from build123d import *

# Parameters (mm, degrees)
SZKIC2_R                   = 2.5
WYTNIJ_WYCI_GNI_CIE1_DEPTH = 102.105666205
ZAOKR_GLENIE1_R            = 10
ZAOKR_GLENIE2_R            = 5
SFAZOWANIE1_SIZE           = 1
SFAZOWANIE2_SIZE           = 0.5
SFAZOWANIE3_SIZE           = 0.5
SZKIC3_R                   = 8
WYTNIJ_WYCI_GNI_CIE2_DEPTH = 100.811551129


with BuildPart() as part:
    # Szkic1 → Obrót1 (revolve)
    with BuildSketch(Plane.XY, mode=Mode.PRIVATE) as obr_t1_sk:
        with BuildLine():
            Line((0, 27.578244749), (0, 21.078244749))
            Line((0, 21.078244749), (-8, 21.078244749))
            Line((-8, 21.078244749), (-8, -8.921755251))
            Line((-8, -8.921755251), (-4, -8.921755251))
            Line((-4, -8.921755251), (-4, -11.921755251))
            Line((-4, -11.921755251), (-8.2, -11.921755251))
            Line((-8.2, -11.921755251), (-8.2, -14.421755251))
            Line((-8.2, -14.421755251), (-10.1, -14.421755251))
            Line((-10.1, -14.421755251), (-10.1, -27.421755251))
            Line((-10.1, -27.421755251), (-20.1, -27.421755251))
            Line((-20.1, -27.421755251), (-20.1, -14.421755251))
            Line((-20.1, -14.421755251), (-12, -3.992443519))
            Line((-12, -3.992443519), (-12, 27.578244749))
            Line((-12, 27.578244749), (-11.5, 27.578244749))
            ThreePointArc((-11.5, 27.578244749), (-11.207862875, 26.874632586), (-10.504874285, 26.580998091))
            Line((-10.504874285, 26.580998091), (-1.498959596, 26.580998091))
            ThreePointArc((-1.498959596, 26.580998091), (-0.793496456, 26.873284267), (-0.5, 27.578244749))
            Line((-0.5, 27.578244749), (0, 27.578244749))
        make_face()
    revolve(obr_t1_sk.sketch.rotate(Axis((-20.1, -27.421755251, 0), (1, 0, 0)), 90), axis=Axis((-20.1, -27.421755251, 0), (1, 0, 0)))

    # Szkic2 → Wytnij-wyciągnięcie1 (cut, through all)
    with BuildSketch(Plane.ZY.offset(20.1)):
        with Locations((0, -27.421755251)):
            Circle(SZKIC2_R)
    extrude(amount=-WYTNIJ_WYCI_GNI_CIE1_DEPTH, mode=Mode.SUBTRACT)

    # Zaokrąglenie1
    zaokr_glenie1_edges = [part.edges().sort_by_distance(p)[0] for p in [
        (-20.1, -27.421755251, -13),
        (-12, -27.421755251, -23.429311732),
    ]]
    fillet(zaokr_glenie1_edges, radius=ZAOKR_GLENIE1_R)

    # Zaokrąglenie2
    zaokr_glenie2_edges = [part.edges().sort_by_distance(p)[0] for p in [
        (0, -27.421755251, -48.5),
    ]]
    fillet(zaokr_glenie2_edges, radius=ZAOKR_GLENIE2_R)

    # Sfazowanie1
    sfazowanie1_edges = [part.edges().sort_by_distance(p)[0] for p in [
        (-10.1, -27.421755251, -2.5),
        (-20.1, -27.421755251, -2.5),
    ]]
    chamfer(sfazowanie1_edges, length=SFAZOWANIE1_SIZE)

    # Sfazowanie2
    sfazowanie2_edges = [part.edges().sort_by_distance(p)[0] for p in [
        (-8.2, -27.421755251, -13),
        (-10.1, -27.421755251, -13),
    ]]
    chamfer(sfazowanie2_edges, length=SFAZOWANIE2_SIZE)

    # Sfazowanie3
    sfazowanie3_edges = [part.edges().sort_by_distance(p)[0] for p in [
        (-4, -27.421755251, -15.5),
        (-8.2, -27.421755251, -15.5),
    ]]
    chamfer(sfazowanie3_edges, length=SFAZOWANIE3_SIZE)

    # Szkic3 → Wytnij-wyciągnięcie2 (cut, through all)
    with BuildSketch(Plane.ZY.offset(12)):
        with Locations((37.829338499, -24.741520982)):
            Circle(SZKIC3_R)
        with Locations((34.101285283, -44.015273535)):
            Circle(SZKIC3_R)
        with Locations((21.235820215, -58.842806265)):
            Circle(SZKIC3_R)
        with Locations((2.68023427, -65.25109375)):
            Circle(SZKIC3_R)
        with Locations((-16.593518284, -61.523040535)):
            Circle(SZKIC3_R)
        with Locations((-31.421051014, -48.657575467)):
            Circle(SZKIC3_R)
        with Locations((-37.829338499, -30.101989521)):
            Circle(SZKIC3_R)
        with Locations((-34.101285283, -10.828236968)):
            Circle(SZKIC3_R)
        with Locations((-21.235820215, 3.999295762)):
            Circle(SZKIC3_R)
        with Locations((-2.68023427, 10.407583248)):
            Circle(SZKIC3_R)
        with Locations((16.593518284, 6.679530032)):
            Circle(SZKIC3_R)
        with Locations((31.421051014, -6.185935036)):
            Circle(SZKIC3_R)
    extrude(amount=-WYTNIJ_WYCI_GNI_CIE2_DEPTH, mode=Mode.SUBTRACT)


solid = part.part
For this review, take the finished solid that the model builds, in its own axes (mm). A direction names the side the tool comes from. Round coordinates to 2 decimals unless told otherwise and drop trailing zeros. Loops run counter-clockwise (first coordinate to the right, second up) from the corner with the lowest first, then second, coordinate; pieces in that order, holes last. Notation, with made-up numbers: (7.25, 64) - (29.25, 64) arc R22 cw to (29.25, 92) - close; hole circle Ø11 at (31.5, -4). An arc over 180 degrees is marked (long way). Use one line per item in the form item = value.
Item 1: Tool access review of faces 3 (the cylindrical face through (-10.028, -40.726, -32.462)), 4 (the cylindrical face through (-6.12, -42.79, -2.02)), 5 (the flat face through (-12, -3.7, 13)): name each direction out of +Z, -Z, +X, -X, +Y, -Y from which nothing blocks a thin tool from reaching the whole face with its end or side.
Answers:
face_3 = +X, -X
face_4 = +X
face_5 = -X
Item 2: For line 1 (X direction, y = -63.5, z = 41); line 2 (Y direction, x = -9.25, z = -15); line 3 (Z direction, x = -9, y = 2), list the stretches that pass through material, from the lowest coordinate up.
Answers:
line_1 = -12 to -11.42, -0.58 to 0
line_2 = -79.3 to -69.36, -53.68 to -1.01, 9.01 to 24.46
line_3 = -45.28 to -28.98, -13.49 to 10.1, 23.08 to 45.28
Item 3: Consider section B-B on x = -15.75. Write out the cut boundary in (y, z).
Answers:
outline = circle Ø37.2 at (-27.42, 0); hole circle Ø5 at (-27.42, 0)
Item 4: Clearance check with flat-ended pins moving along their axes: P1, Ø20, axis at y = -27, z = -2, coming from the +X side; P2, Ø1.5, axis at x = -15.5, z = 2.5, coming from the -Y side; P3, Ø12, axis at y = -49.5, z = 15.5, coming from the +X side. State where each tip first meets the part, or that it passes through.
Answers:
P1 = -10.1
P2 = -47.16
P3 = -8
Item 5: Mouldability with a two-part tool opening along Y and no side actions: class faces 1 (the cylindrical face through (-10.03, -33.17, -30.44)), 2 (the flat face through (0, 25, 12)) as +Y half, -Y half, draft (parallel to the pull), parting line (faces both ways), or undercut.
Answers:
face_1 = undercut
face_2 = draft
Item 6: Consider section A-A on z = 0. State how many separate pieces and enclosed holes the cut face has, then the cut area to 3 significant figures.
Answers:
separate_pieces = 4
enclosed_holes = 0
area = 603 mm^2
